```python
from build123d import *

# Parameters (mm, degrees)
RESSALTO_EXTRUS_O1_DEPTH = 12
CORTE_EXTRUS_O2_REACH    = 15.206
ESBO_O3_R                = 1.5


with BuildPart() as part:
    # Esboço1 → Ressalto-extrusão1 (new body)
    with BuildSketch(Plane.XY):
        Polygon((-0.842772028, 3.952602768), (-3.844440422, 1.246439398), (-3.001668394, -2.70616337), (0.842772028, -3.952602768), (3.844440422, -1.246439398), (3.001668394, 2.70616337), align=None)
    extrude(amount=RESSALTO_EXTRUS_O1_DEPTH)

    # Esboço3 → Corte-extrusão2 (cut, up to next)
    with BuildSketch(Plane(origin=(0, 0, 0), x_dir=(-1, 0, 0), z_dir=(0, 0, -1)), mode=Mode.PRIVATE) as corte_extrus_o2_sk1:
        Circle(ESBO_O3_R)
    corte_extrus_o2_tool1 = extrude(corte_extrus_o2_sk1.sketch, amount=-CORTE_EXTRUS_O2_REACH, mode=Mode.PRIVATE) & part.part
    add(corte_extrus_o2_tool1.solids().sort_by_distance((0, 0, 0))[0], mode=Mode.SUBTRACT)


solid = part.part
```
Design review of the part built by this model. Coordinates are the model's own, in mm. Coordinates: 2 decimals unless noted, no trailing zeros. Loops run counter-clockwise (first coordinate to the right, second up) from the corner with the lowest first, then second, coordinate; pieces in that order, holes last. Notation, with made-up numbers: (-31.5, -13) - (-7.5, -13) arc R24 ccw to (-7.5, 2) - close; hole circle Ø10 at (48, 33). An arc over 180 degrees is marked (long way). Use CSV: the item, a comma, the result in double quotes. Start each with the question number.
1) Consider section A-A on x = -0.5. Write out the cut boundary in (y, z), then the cut area to 3 significant figures.
2) Consider section C-C on y = 0. Write out the cut boundary in (x, z), then the cut area to 3 significant figures.
3) Wall thickness on L1, parallel to X at y = 0.5, z = 10; L2, parallel to Y at x = 0, z = 6.75; L3, parallel to Y at x = -1, z = 10.25: over which ranges is each line inside the solid? List them lowest first. Write a range as from..to.
4) Consider section D-D on y = -3. Write out the cut boundary in (x, z), then the cut area to 3 significant figures.
5) Consider section B-B on z = 10.5. Write out the cut boundary in (x, y).
6) The part is to be moulded in two halves that separate along X. For faces 1 (the flat face through (-1.11, -3.32, 5.92)), 2 (the flat face through (2, 0, 12)), 3 (the cylindrical face through (1.5, 0.07, 5.92)), say which applies: +X half, -X half, draft (parallel to the pull), parting line (faces both ways), or undercut.
7) For pin 1 Ø3 at (y, z) = (-2.5, 7.5) entering from +X, flat-tipped, find the tip position at first contact; note if it passes through.
Geometry says:
1,outline,"(-3.52, 0) - (-1.41, 0) - (-1.41, 12) - (-3.52, 12) - close; (1.41, 0) - (3.84, 0) - (3.84, 12) - (1.41, 12) - close"
1,area,"54.4 mm^2"
2,outline,"(-3.58, 0) - (-1.5, 0) - (-1.5, 12) - (-3.58, 12) - close; (1.5, 0) - (3.58, 0) - (3.58, 12) - (1.5, 12) - close"
2,area,"49.9 mm^2"
3,L1,"-3.69..-1.41, 1.41..3.47"
3,L2,"-3.68..-1.5, 1.5..3.68"
3,L3,"-3.36..-1.12, 1.12..3.81"
4,outline,"(-2.1, 0) - (1.9, 0) - (1.9, 12) - (-2.1, 12) - close"
4,area,"47.9 mm^2"
5,outline,"(-3.84, 1.25) - (-3, -2.71) - (0.84, -3.95) - (3.84, -1.25) - (3, 2.71) - (-0.84, 3.95) - close; hole circle Ø3 at (0, 0)"
6,face 1,"-X half"
6,face 2,"draft"
6,face 3,"undercut"
7,pin 1,"x = 3.84"
